Model file for the job. Use its own axes, mm. A direction names the side the tool comes from. Give positions to 0.01 mm unless a question says otherwise; leave off trailing zeros. Loops run counter-clockwise (first coordinate to the right, second up) from the corner with the lowest first, then second, coordinate; pieces in that order, holes last. Notation, with made-up numbers: (80.25, -11) - (134.25, -11) arc R7 ccw to (134.25, -5) - close; hole circle Ø8 at (0.25, -21). An arc over 180 degrees is marked (long way). Use a Markdown table: item, result.
from build123d import *

# Parameters (mm, degrees)
SKETCH2_W           = 203.2
SKETCH2_H           = 101.6
BOSS_EXTRUDE1_DEPTH = 19.558
SKETCH3_W           = 76.2
SKETCH3_H           = 5.08
CUT_EXTRUDE2_DEPTH  = 19.558
FILLET1_R           = 10
FILLET2_R           = 10
FILLET3_R           = 10
FILLET4_R           = 10
EXTRUDE_THIN5_DEPTH = 25.4


with BuildPart() as part:
    # Sketch2 → Boss-Extrude1 (new body)
    with BuildSketch(Plane(origin=(-97.482495003, 0, 34.735141898), x_dir=(1, 0, 0), z_dir=(0, 1, 0))):
        with Locations((-19.545959724, 34.347881976)):
            Rectangle(SKETCH2_W, SKETCH2_H)
    extrude(amount=BOSS_EXTRUDE1_DEPTH)

    # Sketch3 → Cut-Extrude2 (cut)
    with BuildSketch(Plane(origin=(-97.482495003, 19.558, 34.735141898), x_dir=(1, 0, 0), z_dir=(0, 1, 0))):
        Polygon((48.044591515, 85.147881976), (-28.155408485, 85.147881976), (-28.155408485, 69.907881976), (-15.015206922, 69.907881976), (2.604442641, 69.907881976), (2.604442641, 63.303881976), (22.924442641, 63.303881976), (22.924442641, 69.907881976), (48.044591515, 69.907881976), align=None)
        with Locations((9.944591515, 87.687881976)):
            Rectangle(SKETCH3_W, SKETCH3_H)
    cut_extrude2 = extrude(amount=-CUT_EXTRUDE2_DEPTH, mode=Mode.SUBTRACT)

    # Mirror4: Cut-Extrude2 across plane
    add(cut_extrude2.mirror(Plane.XY), mode=Mode.SUBTRACT)

    # Fillet1
    fillet1_edges = [part.edges().sort_by_distance(p)[0] for p in [
        (-15.428454726, 9.779, 51.187259921),
    ]]
    fillet(fillet1_edges, radius=FILLET1_R)

    # Fillet2
    fillet2_edges = [part.edges().sort_by_distance(p)[0] for p in [
        (-218.628454726, 9.779, -50.412740079),
    ]]
    fillet(fillet2_edges, radius=FILLET2_R)

    # Fillet3
    fillet3_edges = [part.edges().sort_by_distance(p)[0] for p in [
        (-218.628454726, 9.779, 51.187259921),
    ]]
    fillet(fillet3_edges, radius=FILLET3_R)

    # Fillet4
    fillet4_edges = [part.edges().sort_by_distance(p)[0] for p in [
        (-15.428454726, 9.779, -50.412740079),
    ]]
    fillet(fillet4_edges, radius=FILLET4_R)

    # Sketch7 → Extrude-Thin5 (add)
    with BuildSketch(Plane(origin=(0, 19.558, 0), x_dir=(1, 0, 0), z_dir=(0, 1, 0))):
        Polygon((-132.522454726, 50.412740079), (-132.522454726, 20.948740079), (-15.428454726, 20.948740079), (-15.428454726, 18.408740079), (-135.062454726, 18.408740079), (-135.062454726, 50.412740079), align=None)
    extrude_thin5 = extrude(amount=EXTRUDE_THIN5_DEPTH)

    # Mirror5: Extrude-Thin5 across plane
    add(extrude_thin5.mirror(Plane.XY))


solid = part.part
(1) Slice it at B-B, the plane y = 37. Write the cut outline in (x, z), plus the area to 3 significant figures.
Computed:
| item | result |
|---|---|
| outline | (-135.06, -50.41) - (-132.52, -50.41) - (-132.52, -20.95) - (-15.43, -20.95) - (-15.43, -18.41) - (-135.06, -18.41) - close; (-135.06, 18.41) - (-15.43, 18.41) - (-15.43, 20.95) - (-132.52, 20.95) - (-132.52, 50.41) - (-135.06, 50.41) - close |
| area | 757 mm² |
(2) Mould opens along X. For faces 6 (the flat face through (-132.522, 32, -36)), 7 (the flat face through (-62, 19.558, -33)), 8 (the flat face through (-62, 10, -35.173)) say: pulls with the +X half, pulls with the -X half, needs draft (parallel to the pull), parting line crosses it, or undercut.
Computed:
| item | result |
|---|---|
| face 6 | pulls with the +X half |
| face 7 | needs draft |
| face 8 | undercut |
(3) 3-axis set-ups, long thin cutter, end or side, ignore diameter. For faces 1 (the flat face through (-110, 10, -35.173)), 2 (the cylindrical face through (-215.777, 9.916, 48.18)), 3 (the flat face through (-94.878, 10, 32)), 4 (the flat face through (-74, 32, 18.409)), 5 (the flat face through (-132.522, 32, 36)): which of +Z, -Z, +X, -X, +Y, -Y reach the whole face in a straight line?
Computed:
| item | result |
|---|---|
| face 1 | -Z, +Y, -Y |
| face 2 | +Z, -X, +Y, -Y |
| face 3 | +Z, +Y, -Y |
| face 4 | +X, -X, +Y |
| face 5 | +Z, +X, +Y |
(4) Pin check, flat tips, straight feed: P1, Ø10, axis at x = -58.5, y = 39, coming from the -Z side; P2, Ø0.8, axis at x = -134, y = 38.5, coming from the +Z side; P3, Ø6, axis at x = -86, y = 6.5, coming from the +Z side; P4, Ø20.5, axis at y = 29.5, z = 37.5, coming from the +X side. Stop position of each tip, or through.
Computed:
| item | result |
|---|---|
| P1 | z = -20.95 |
| P2 | z = 50.41 |
| P3 | z = 28.57 |
| P4 | x = -15.43 |
(5) Drill centre lines: probe 1 along X at (y, z) = (19.5, -32); probe 2 along Z at (x, y) = (-43, 32.5); probe 3 along Y at (x, z) = (-165.5, 27). Where is each one in solid material? Low to high. Write a range as [from, to].
Computed:
| item | result |
|---|---|
| probe 1 | [-218.63, -94.88], [-74.56, -15.43] |
| probe 2 | [-20.95, -18.41], [18.41, 20.95] |
| probe 3 | [0, 19.56] |
(6) Slice it at D-D, the plane y = 7.5. Write the cut outline in (x, z), plus the area to 3 significant figures.
Computed:
| item | result |
|---|---|
| outline | (-218.63, -40.41) arc R10 ccw to (-208.63, -50.41) - (-125.64, -50.41) - (-125.64, -35.17) - (-94.88, -35.17) - (-94.88, -28.57) - (-74.56, -28.57) - (-74.56, -35.17) - (-49.44, -35.17) - (-49.44, -50.41) - (-25.43, -50.41) arc R10 ccw to (-15.43, -40.41) - (-15.43, 41.19) arc R10 ccw to (-25.43, 51.19) - (-49.44, 51.19) - (-49.44, 35.17) - (-74.56, 35.17) - (-74.56, 28.57) - (-94.88, 28.57) - (-94.88, 35.17) - (-125.64, 35.17) - (-125.64, 51.19) - (-208.63, 51.19) arc R10 ccw to (-218.63, 41.19) - close |
| area | 17,900 mm² |
(7) Slice it at A-A, the plane x = -51.5. Write the cut outline in (y, z).
Computed:
| item | result |
|---|---|
| outline | (0, -35.17) - (19.56, -35.17) - (19.56, -20.95) - (44.96, -20.95) - (44.96, -18.41) - (19.56, -18.41) - (19.56, 18.41) - (44.96, 18.41) - (44.96, 20.95) - (19.56, 20.95) - (19.56, 35.17) - (0, 35.17) - close |
(8) Slice it at C-C, the plane z = -30.5. Write the cut outline in (x, y).
Computed:
| item | result |
|---|---|
| outline | (-218.63, 0) - (-94.88, 0) - (-94.88, 19.56) - (-132.52, 19.56) - (-132.52, 44.96) - (-135.06, 44.96) - (-135.06, 19.56) - (-218.63, 19.56) - close; (-74.56, 0) - (-15.43, 0) - (-15.43, 19.56) - (-74.56, 19.56) - close |
